Geometry check sheet. Reference: the model listing, model coordinates, mm. Face numbers are marked on the shaded views. A direction names the side the tool comes from. Give positions to 0.01 mm unless a question says otherwise; leave off trailing zeros. Loops run counter-clockwise (first coordinate to the right, second up) from the corner with the lowest first, then second, coordinate; pieces in that order, holes last. Notation, with made-up numbers: (75.5, -12.5) -> (79.5, -12.5) arc R23 cw to (79.5, 6.5) -> close; hole circle Ø3 at (51.25, 59.5). An arc over 180 degrees is marked (long way). Write each question's results on one line, items separated by ' | '. Start each with the question number.
1) Sectioned sample at B-B on x = 8.5. Record the cut outline in (y, z).
2) Depth check by flat-ended pin: pin 1 (4 mm diameter, centred on x = 67.5, z = 46, fed in from +Y); pin 2 (1.3 mm diameter, centred on x = -2, y = 12.5, fed in from -Z); pin 3 (2.5 mm diameter, centred on x = 15.5, z = 2.5, fed in from +Y); pin 4 (0.5 mm diameter, centred on x = -2, y = 9.5, fed in from -Z). Enter the tip coordinate at first touch or a pass-through.
3) Set-up check for the marked faces 1 and 2: record each of +Z, -Z, +X, -X, +Y, -Y from which the full face is reachable in a straight line by a thin tool's end or side.
4) Draft check along X on the marked faces 3, 4 and 5. Enter one of: pulls with the +X half, pulls with the -X half, needs draft (parallel to the pull), parting line crosses it, or undercut.
5) Scan lines: line 1 (Z direction, x = 66.04, y = 1.75) (1 decimal); line 2 (X direction, y = 22.75, z = 39); line 3 (Z direction, x = 60, y = 7). Record each from-to range of solid material in increasing order. Write a range as from..to.
6) Sectioned sample at C-C on z = 45.72. Count the separate pieces of the cut face and the enclosed holes in it, then the cut area to 3 significant figures.
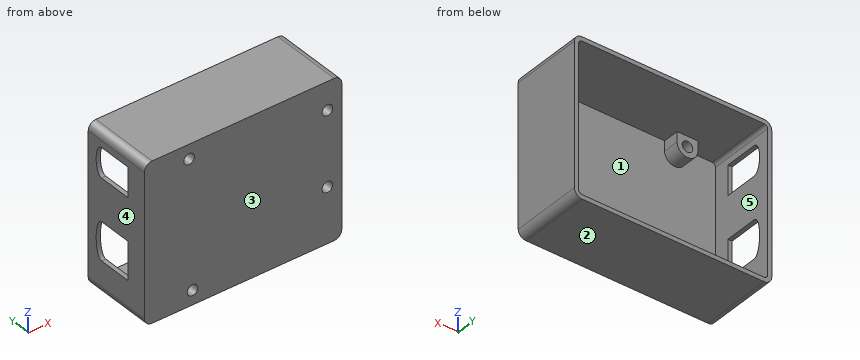
Autodesk Inventor part; units mm, degrees
ref_plane "YZ Plane" through (0, 0, 0) normal (1, 0, 0) x (0, 1, 0)
ref_plane "XZ Plane" through (0, 0, 0) normal (0, 1, 0) x (-1, 0, 0)
ref_plane "XY Plane" through (0, 0, 0) normal (0, 0, 1) x (1, 0, 0)
sketch "Sketch1" plane through (0, 0, 0) normal (0, 1, 0) x (-1, 0, 0)
  circle A0 centre (-15.24, 2.54) radius 2
  circle A1 centre (-66.04, 17.78) radius 2
  circle A2 centre (-66.04, 45.72) radius 2
  line L0 (0, 0) -> (-68.58, 0) construction
  line L1 (-68.58, 0) -> (-68.58, 53.34) construction
  line L2 (-68.58, 53.34) -> (0, 53.34) construction
  line L3 (0, 53.34) -> (0, 0) construction
  line L4 (-68.58, -1.27) -> (0, -1.27)
  line L5 (1.27, 0) -> (1.27, 53.34)
  line L6 (0, 54.61) -> (-68.58, 54.61)
  line L7 (-69.85, 53.34) -> (-69.85, 0)
  arc A3 (0, -1.27) -> (1.27, 0) centre (0, 0) ccw
  arc A4 (-69.85, 0) -> (-68.58, -1.27) centre (-68.58, 0) ccw
  arc A5 (-68.58, 54.61) -> (-69.85, 53.34) centre (-68.58, 53.34) ccw
  arc A6 (1.27, 53.34) -> (0, 54.61) centre (0, 53.34) ccw
  arc A7 (-11.335, 2.54) -> (-19.145, 2.54) centre (-15.24, 2.54) ccw
  arc A8 (-66.04, 41.815) -> (-66.04, 49.625) centre (-66.04, 45.72) ccw
  arc A9 (-66.04, 13.875) -> (-66.04, 21.685) centre (-66.04, 17.78) ccw
  line L8 (-11.335, 2.54) -> (-19.145, 2.54) construction
  line L9 (-19.145, 2.54) -> (-19.145, -1.27)
  line L10 (-19.145, -1.27) -> (-11.335, -1.27)
  line L11 (-11.335, -1.27) -> (-11.335, 2.54)
  line L12 (-66.04, 13.875) -> (-69.85, 13.875)
  line L13 (-69.85, 13.875) -> (-69.85, 21.685)
  line L14 (-69.85, 21.685) -> (-66.04, 21.685)
  line L15 (-66.04, 21.685) -> (-66.04, 13.875) construction
  line L16 (-66.04, 41.815) -> (-69.85, 41.815)
  line L17 (-69.85, 41.815) -> (-69.85, 49.625)
  line L18 (-69.85, 49.625) -> (-66.04, 49.625)
  line L19 (-66.04, 49.625) -> (-66.04, 41.815) construction
  line L20 (-11.335, 54.61) -> (-19.145, 54.61)
  circle A10 centre (-13.97, 50.8) radius 2
  circle A11 centre (-13.97, 50.8) radius 3.905 construction
  arc A12 (-17.875, 50.8) -> (-10.065, 50.8) centre (-13.97, 50.8) ccw
  line L21 (-17.875, 50.8) -> (-17.875, 54.61)
  line L22 (-10.065, 50.8) -> (-10.065, 54.61)
  point P0 (-15.24, 2.54)
  dimension "d0" = 4
  dimension "d4" = 15.24
  dimension "d5" = 2.54
  dimension "d6" = 17.78
  dimension "d7" = 66.04
  dimension "d8" = 45.72
  dimension "d10" = 2.54
  dimension "d12" = 1.27
  dimension "d13" = 1.27
  dimension "d14" = 1.905
  dimension "d51" = 53.34
  dimension "d52" = 50.8
  dimension "d54" = 1.27
extrude "Extrusion1" add sketch "Sketch1" along normal blind 6 contours L9 A7 L11 L4 | L7 L14 A9 L12 | L7 L18 A8 L16 | L22 A12 L21 L6
extrude "Extrusion2" add sketch "Sketch1" against normal blind 2
sketch "Sketch2" plane through (0, -2, 0) normal (0, -1, 0) x (1, 0, 0)
  line L0 (68.58, 54.61) -> (0, 54.61)
  arc A0 (0, 54.61) -> (-1.27, 53.34) centre (0, 53.34) ccw
  line L1 (-1.27, 53.34) -> (-1.27, 0)
  arc A1 (-1.27, 0) -> (0, -1.27) centre (0, 0) ccw
  line L2 (0, -1.27) -> (68.58, -1.27)
  arc A2 (68.58, -1.27) -> (69.85, 0) centre (68.58, 0) ccw
  line L3 (69.85, 0) -> (69.85, 53.34)
  arc A3 (69.85, 53.34) -> (68.58, 54.61) centre (68.58, 53.34) ccw
  line L4 (68.58, -2.8575) -> (0, -2.8575)
  arc A4 (-2.8575, 0) -> (0, -2.8575) centre (0, 0) ccw
  line L5 (-2.8575, 0) -> (-2.8575, 53.34)
  arc A5 (0, 56.1975) -> (-2.8575, 53.34) centre (0, 53.34) ccw
  line L6 (0, 56.1975) -> (68.58, 56.1975)
  arc A6 (71.4375, 53.34) -> (68.58, 56.1975) centre (68.58, 53.34) ccw
  line L7 (71.4375, 53.34) -> (71.4375, 0)
  arc A7 (68.58, -2.8575) -> (71.4375, 0) centre (68.58, 0) ccw
  point P0 (0, 0)
  dimension "d19" = 1.5875
extrude "Extrusion3" add sketch "Sketch2" against normal blind 27.05
sketch "Sketch4" plane through (-2.8575, -2, 0) normal (-1, 0, 0) x (0, 0, 1)
  line L0 (0, 2) -> (53.34, 2)
  line L1 (0, 27.05) -> (53.34, 27.05)
  line L2 (50.8, 20.7) -> (39.6875, 20.7) construction
  line L3 (39.6875, 20.7) -> (39.6875, 8)
  ellipse E0 centre (45.2438, 20.7) end of major axis (50.8, 20.7) minor radius 2.54 (50.8, 20.7) -> (39.6875, 20.7) ccw
  ellipse E1 centre (45.2438, 20.7) end of major axis (50.8, 20.7) minor radius 2.54 (39.6875, 20.7) -> (50.8, 20.7) ccw construction
  line L4 (9.525, 8) -> (9.525, 20.7)
  line L5 (23.8125, 8) -> (23.8125, 20.7)
  ellipse E2 centre (16.6688, 20.7) end of major axis (23.8125, 20.7) minor radius 2.54 (23.8125, 20.7) -> (9.525, 20.7) ccw
  line L6 (9.525, 8) -> (23.8125, 8)
  line L7 (50.8, 20.7) -> (50.8, 8)
  line L8 (50.8, 8) -> (39.6875, 8)
  line L9 (50.8, 8) -> (54.61, 8)
  line L10 (54.61, 8) -> (50.8, 8)
  line L11 (50.8, 8) -> (50.8, 8)
  line L12 (48.8, 8) -> (52.8, 8)
  line L13 (2.54, 8) -> (-1.27, 8)
  line L14 (-1.27, 8) -> (2.54, 8)
  line L15 (2.54, 8) -> (2.54, 8)
  line L16 (0.54, 8) -> (4.54, 8)
  line L17 (53.34, 0) -> (53.34, 27.05)
  point P0 (2.54, 2)
  point P1 (2.54, 2)
  point P2 (2.54, 2)
  point P3 (2.54, 2)
  dimension "d26" = 2.54
  dimension "d29" = 2.54
  dimension "d25" = 11.1125
  dimension "d27" = 9.525
  dimension "d28" = 14.2875
  dimension "d56" = 2.54
  dimension "d57" = 12.7
extrude "Extrusion5" cut sketch "Sketch4" against normal up to surface (1.5875 mm away)
sketch "Sketch6" plane through (0, 0, 0) normal (0, 1, 0) x (1, 0, 0)
  line L0 (28.6568, -13.7506) -> (43.0772, -34.6602)
  point P0 (0, 0)
  dimension "d50" = 25.4
sketch "Sketch7" plane through (-2.8575, -2, 0) normal (-1, 0, 0) x (0, 0, 1)
  line L0 (0, 0) -> (0, 27.05)
  line L1 (0, 0) -> (-8.89, 0)
  line L2 (-8.89, 0) -> (-21.1351, -14.5931)
  line L3 (-21.1351, -14.5931) -> (-21.1351, -17.1331)
  line L4 (-21.1351, -17.1331) -> (11.9427, -44.8887)
  line L5 (53.34, 0) -> (0, 0) construction
  line L6 (26.67, 0) -> (26.67, -45.2204) construction
  line L7 (-8.89, 0) -> (25.1607, -28.5719) construction
  point P0 (0, 2)
  dimension "d58" = 8.89
  dimension "d59" = 19.05
  dimension "d60" = 130
  dimension "d61" = 2.54
  dimension "d62" = 43.18
  dimension "d63" = 130
properties part number "ArduinoHolder-v2"
Result:
1) outline: (-2, -2.86) -> (25.05, -2.86) -> (25.05, -1.27) -> (0, -1.27) -> (0, 54.61) -> (25.05, 54.61) -> (25.05, 56.2) -> (-2, 56.2) -> close
2) pin 1: y = 6 | pin 2: z = -2.52 | pin 3: through | pin 4: z = -2.26
3) face 1: +Y | face 2: -Z, +X, -X, +Y, -Y
4) face 3: needs draft | face 4: pulls with the -X half | face 5: undercut
5) line 1: -2.9..-1.3, 13.9..15.8, 19.8..21.7, 41.8..43.7, 47.7..49.6, 54.6..56.2 | line 2: -2.86..-1.27, 69.85..71.44 | line 3: -2.86..-1.27, 54.61..56.2
6) separate pieces: 3 | enclosed holes: 0 | area: 218 mm^2
